Here's the drawing with two shaded views (mm, measured from the low corner). I have some questions. Round coordinates to 2 decimals unless told otherwise and drop trailing zeros. Loops run counter-clockwise (first coordinate to the right, second up) from the corner with the lowest first, then second, coordinate; pieces in that order, holes last. Notation, with made-up numbers: (38.25, 50) -> (52.25, 50) arc R7 ccw to (52.25, 62) -> close; hole circle Ø1 at (52, 57). An arc over 180 degrees is marked (long way). Write each question's results on one line, items separated by ' | '.
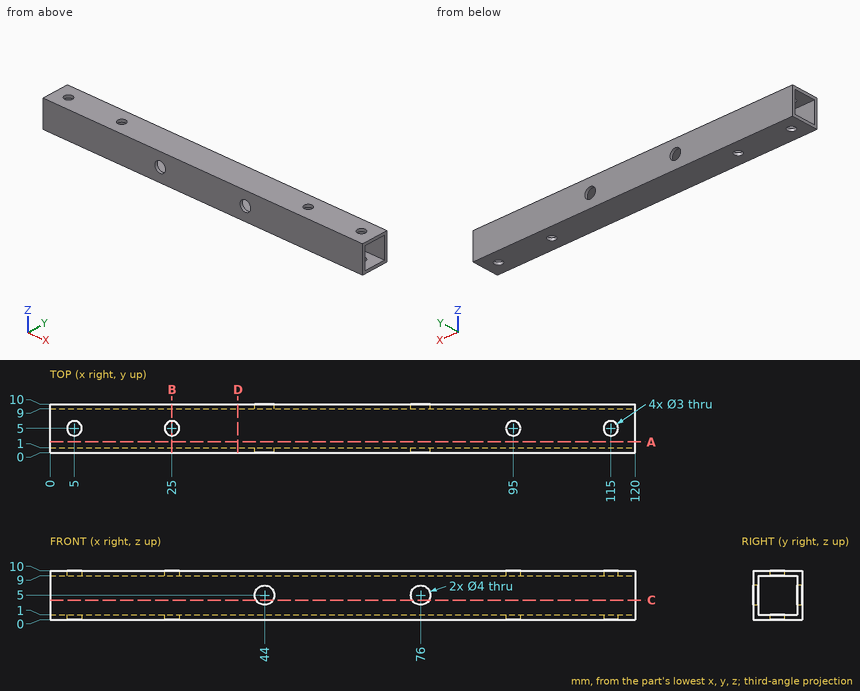
1. If we section it at A-A (y = 2.25): List the corners of the cut face in (x, z) for me.
Final values:
outline: (0, 0) -> (120, 0) -> (120, 1) -> (0, 1) -> close; (0, 9) -> (120, 9) -> (120, 10) -> (0, 10) -> close
2. If we section it at D-D (x = 38.5): List the corners of the cut face in (y, z) for me.
Final values:
outline: (0, 0) -> (10, 0) -> (10, 10) -> (0, 10) -> close; hole (1, 1) -> (9, 1) -> (9, 9) -> (1, 9) -> close
3. If we section it at C-C (z = 4): List the corners of the cut face in (x, y) for me.
Final values:
outline: (0, 0) -> (42.27, 0) -> (42.27, 1) -> (0, 1) -> close; (0, 9) -> (42.27, 9) -> (42.27, 10) -> (0, 10) -> close; (45.73, 0) -> (74.27, 0) -> (74.27, 1) -> (45.73, 1) -> close; (45.73, 9) -> (74.27, 9) -> (74.27, 10) -> (45.73, 10) -> close; (77.73, 0) -> (120, 0) -> (120, 1) -> (77.73, 1) -> close; (77.73, 9) -> (120, 9) -> (120, 10) -> (77.73, 10) -> close
4. If we section it at B-B (x = 25): List the corners of the cut face in (y, z) for me.
Final values:
outline: (0, 0) -> (3.5, 0) -> (3.5, 1) -> (1, 1) -> (1, 9) -> (3.5, 9) -> (3.5, 10) -> (0, 10) -> close; (6.5, 0) -> (10, 0) -> (10, 10) -> (6.5, 10) -> (6.5, 9) -> (9, 9) -> (9, 1) -> (6.5, 1) -> close
5. Please list where these lines run through material, in increasing order: line 1 (X direction, y = 0.7, z = 5); line 2 (Y direction, x = 28, z = 3.25). Write a range as from..to.
Final values:
line 1: 0..42, 46..74, 78..120 | line 2: 0..1, 9..10
